CAD build for the part. Positions are in the model's coordinates, mm. Give positions to 0.01 mm unless a question says otherwise; leave off trailing zeros. Loops run counter-clockwise (first coordinate to the right, second up) from the corner with the lowest first, then second, coordinate; pieces in that order, holes last.
```python
from build123d import *

# Parameters (mm, degrees)
F0_R     = 12.5
F3_W     = 28.4879058599
F3_H     = 25.5846790969
F4_DEPTH = 25


with BuildPart() as f2:
    # F2: sweep along a path in F1
    with BuildLine(Plane.XZ) as f2_path:
        add(Plane.XZ * Edge.make_bspline(
            [(-52.7663948565, -36.1680299247), (-34.8857263736, -17.9429488086), (0.1127210252, 17.7296292828), (31.7565659621, -17.5018500525), (47.2336051435, -34.7336051435)],
            knots=[0, 0, 0, 0, 0.5108989059, 1, 1, 1, 1], degree=3))
    # F0 (on Right) → F2 (sweep)
    with BuildSketch(Plane.YZ):
        Circle(F0_R)
    sweep(path=f2_path.line)

    # F3 (on Top) → F4 (join)
    with BuildSketch(Plane.XY):
        with Locations((0.3629028797, 0.1814505085)):
            Rectangle(F3_W, F3_H)
    extrude(amount=F4_DEPTH)


solid = f2.part
```
1. Drop flat-ended pins along their axis: pin 1 (7.5 mm diameter, centred on y = -6, z = 14.5, fed in from -X); pin 2 (2 mm diameter, centred on y = 1, z = 1, fed in from +X); pin 3 (3 mm diameter, centred on x = 19, y = 1.5, fed in from -Z). Give the stop position or say it passes through.
Responses:
pin 1: stops at x = -13.88
pin 2: stops at x = 30.13
pin 3: stops at z = -24.56
2. Saw through at A-A, the plane z = 20. List the corners of the cut face in (x, y).
Responses:
outline: (-13.88, -12.61) - (14.61, -12.61) - (14.61, 12.97) - (-13.88, 12.97) - close
3. Probe line 1 along Y through (x, z) = (-36, -20); line 2 along X through (y, z) = (5.5, -13); line 3 along X through (y, z) = (2, -35). List the from-to ranges inside material, lowest first.
Responses:
line 1: y = -12.5 to 12.5
line 2: x = -45.36 to -7.84, 6.72 to 42.45
line 3: x = -54 to -34.23, 30.83 to 46.95
